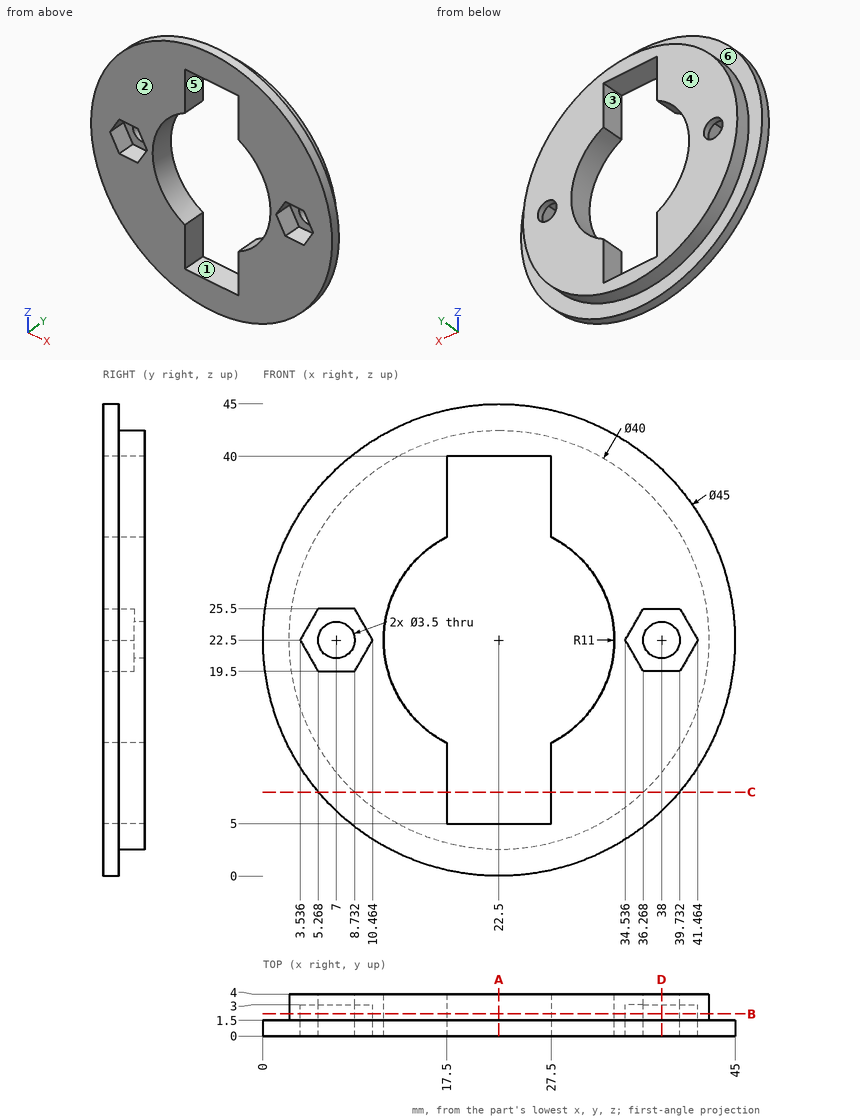
Geometry check sheet. Reference: drawing and pictorial views, mm from the part's lowest x, y, z. A direction names the side the tool comes from. Give positions to 0.01 mm unless a question says otherwise; leave off trailing zeros. Order: outer loops, then holes, each group sorted by start corner. A loop starts at its lowest first (then second) coordinate and runs counter-clockwise, first axis right, second up. Notation, with made-up numbers: (-38, -37) -> (19, -37) arc R16 cw to (19, -20) -> close; hole circle Ø6 at (-1.75, 37). An arc over 180 degrees is marked (long way). Use CSV: the item, a comma, the result in double quotes. Start each with the question number.
1) Sectioned sample at B-B, the plane y = 2.1. Record the boundary of the cut face in (x, z).
2) Go/stop test with flat-tipped pins: P1, Ø1.8, axis at x = 6.5, z = 24, coming from the -Y side; P2, Ø1.2, axis at y = 2, z = 37, coming from the -X side; P3, Ø0.9, axis at x = 39, y = 1.5, coming from the -Z side; P4, Ø3, axis at x = 38, z = 22.5, coming from the -Y side. Record where each tip stops, or that it passes through.
3) Sectioned sample at C-C, the plane z = 8. Record the boundary of the cut face in (x, y) (1 decimal).
4) Mould release check, pull along X, two halves, no side actions. Record for the marked faces 1, 2 and 3: released by +X, released by -X, zero draft, split by the parting line, or undercut.
5) Material ranges on line 1 (Z direction, x = 23, y = 3.3); line 2 (Y direction, x = 3.5, z = 15.5); line 3 (X direction, y = 3.6, z = 9.5), recorded low to high. Write a range as from..to.
6) Set-up check for the marked faces 4, 5 and 6: record each of +Z, -Z, +X, -X, +Y, -Y from which the full face is reachable in a straight line by a thin tool's end or side.
7) Sectioned sample at A-A, the plane x = 22.5. Record the boundary of the cut face in (y, z), plus the area to 3 significant figures.
8) Sectioned sample at D-D, the plane x = 38. Record the boundary of the cut face in (y, z), plus the area to 3 significant figures.
Recorded:
1,outline,"circle Ø40 at (22.5, 22.5); hole (3.54, 22.5) -> (5.27, 19.5) -> (8.73, 19.5) -> (10.46, 22.5) -> (8.73, 25.5) -> (5.27, 25.5) -> close; hole (17.5, 5) -> (27.5, 5) -> (27.5, 12.7) arc R11 ccw to (27.5, 32.3) -> (27.5, 40) -> (17.5, 40) -> (17.5, 32.3) arc R11 ccw to (17.5, 12.7) -> close; hole (34.54, 22.5) -> (36.27, 19.5) -> (39.73, 19.5) -> (41.46, 22.5) -> (39.73, 25.5) -> (36.27, 25.5) -> close"
2,P1,"y = 3"
2,P2,"x = 5.02"
2,P3,"z = 6.73"
2,P4,"through"
3,outline,"(5.3, 0) -> (17.5, 0) -> (17.5, 4) -> (8.7, 4) -> (8.7, 1.5) -> (5.3, 1.5) -> close; (27.5, 0) -> (39.7, 0) -> (39.7, 1.5) -> (36.3, 1.5) -> (36.3, 4) -> (27.5, 4) -> close"
4,face 1,"undercut"
4,face 2,"zero draft"
4,face 3,"undercut"
5,line 1,"2.51..5, 40..42.49"
5,line 2,"0..1.5"
5,line 3,"7.3..17.5, 27.5..37.7"
6,face 4,"+Z, -Z, +X, -X, +Y"
6,face 5,"+Y, -Y"
6,face 6,"+Y"
7,outline,"(0, 0) -> (1.5, 0) -> (1.5, 2.5) -> (4, 2.5) -> (4, 5) -> (0, 5) -> close; (0, 40) -> (4, 40) -> (4, 42.5) -> (1.5, 42.5) -> (1.5, 45) -> (0, 45) -> close"
7,area,"27.5 mm2"
8,outline,"(0, 6.19) -> (1.5, 6.19) -> (1.5, 9.86) -> (4, 9.86) -> (4, 20.75) -> (3, 20.75) -> (3, 19.5) -> (0, 19.5) -> close; (0, 25.5) -> (3, 25.5) -> (3, 24.25) -> (4, 24.25) -> (4, 35.14) -> (1.5, 35.14) -> (1.5, 38.81) -> (0, 38.81) -> close"
8,area,"90.6 mm2"
